Verification items for the finished model (mm, model axes). A direction names the side the tool comes from. Give positions to 0.01 mm unless a question says otherwise; leave off trailing zeros. Write item = value, one per line.
from build123d import *

# Parameters (mm, degrees)
SKETCH1_W               = 100
SKETCH1_H               = 10
BOSS_EXTRUDE1_DEPTH     = 100
ENL_V_MAT_EXTRU_1_DEPTH = 10
CONG_1_R                = 5
CONG_3_R                = 5


with BuildPart() as part:
    # Sketch1 → Boss-Extrude1 (new body)
    with BuildSketch(Plane.XY):
        with Locations((50, 5)):
            Rectangle(SKETCH1_W, SKETCH1_H)
    extrude(amount=BOSS_EXTRUDE1_DEPTH)

    # Esquisse1 → Enlèv. mat.-Extru.1 (cut)
    with BuildSketch(Plane.XZ):
        Polygon((18, 10), (18, 0), (22, 0), (22, 10), (23.55, 10), (23.55, 15.5), (22, 15.5), (22, 21.5), (18, 21.5), (18, 15.5), (16.45, 15.5), (16.45, 10), align=None)
        Polygon((78, 10), (78, 0), (82, 0), (82, 10), (83.55, 10), (83.55, 15.5), (82, 15.5), (82, 21.5), (78, 21.5), (78, 15.5), (76.45, 15.5), (76.45, 10), align=None)
    extrude(amount=-ENL_V_MAT_EXTRU_1_DEPTH, mode=Mode.SUBTRACT)

    # Congé1
    cong_1_edges = [part.edges().sort_by_distance(p)[0] for p in [
        (0, 5, 100),
    ]]
    fillet(cong_1_edges, radius=CONG_1_R)

    # Congé3
    cong_3_edges = [part.edges().sort_by_distance(p)[0] for p in [
        (100, 5, 100),
    ]]
    fillet(cong_3_edges, radius=CONG_3_R)


solid = part.part
1) Tool access check on faces 4 (the flat face through (49, 10, 49)), 5 (the flat face through (18, 5, 19)), 6 (the flat face through (83.55, 5, 13)). Record the directions out of +Z, -Z, +X, -X, +Y, -Y that give a thin tool (end or side, any length) a straight path to the whole face; none if there is none.
From the geometry:
face_4 = +Z, -Z, +X, -X, +Y
face_5 = -Z, +Y, -Y
face_6 = +Y, -Y
2) Depth check by flat-ended pin: P1, Ø6, axis at x = 59.5, y = 1.5, coming from the -Z side. Enter the tip coordinate at first touch or a pass-through.
From the geometry:
P1 = 0
3) Draft check along Z on faces 1 (the flat face through (78, 5, 19)), 2 (the flat face through (80, 5, 21.5)), 3 (the flat face through (16.45, 5, 13)). Enter one of: +Z half, -Z half, draft (parallel to the pull), parting line (faces both ways), or undercut.
From the geometry:
face_1 = draft
face_2 = -Z half
face_3 = undercut
4) Material ranges on probe 1 along X at (y, z) = (8, 4.5); probe 2 along X at (y, z) = (4.75, 11); probe 3 along Z at (x, y) = (79, 6), recorded low to high. Write a range as from..to.
From the geometry:
probe_1 = 0..18, 22..78, 82..100
probe_2 = 0..16.45, 23.55..76.45, 83.55..100
probe_3 = 21.5..100
